Can you work these out from the model? Positions are in its coordinate system, mm. Face numbers are marked on the shaded views. A direction names the side the tool comes from. Round coordinates to 2 decimals unless told otherwise and drop trailing zeros. Write each loop counter-clockwise with the first axis right and the second up, starting at its lowest first coordinate (ties: lowest second). Pieces come first, ordered by that corner, then holes. Notation, with made-up numbers: (37.5, 54.5) - (51.5, 54.5) arc R24 ccw to (51.5, 69.5) - close; hole circle Ø7 at (43, -30). An arc over 180 degrees is marked (long way). One line per item, written item: value. Start each with the question number.
(1) Thinking about a two-plate mould opening in Z: for the marked faces 5, 6 and 7, which applies, +Z half, -Z half, draft (parallel to the pull), parting line (faces both ways), or undercut?
(2) I want a section at D-D on x = 3.75. List the corners of the cut face in (y, z) for me, plus the area to 3 significant figures.
(3) On a 3-axis mill with a long thin cutter (end or side, diameter ignored), from which of +Z, -Z, +X, -X, +Y, -Y can I reach the whole of each face in a straight line? I mean the marked faces 1, 2, 3 and 4. Say none if no direction works.
(4) I want a section at B-B on y = 7.5. List the corners of the cut face in (x, z) for me.
(5) I'm going to push flat-ended pins straight in: pin 1 Ø2 at (x, z) = (0.5, 3) entering from -Y; pin 2 Ø4.5 at (y, z) = (6, 6) entering from -X; pin 3 Ø3 at (x, z) = (10, 7) entering from +Y; pin 4 Ø1.5 at (x, y) = (-2.5, 1.5) entering from +Z. Where does each tip first touch, or does it pass through?
(6) I want a section at A-A on z = 5.75. List the corners of the cut face in (x, y) for me.
(7) If I drill on L1, parallel to X at y = 1.8, z = 5.75; L2, parallel to Z at x = 12, y = 1.8; L3, parallel to X at y = 4, z = 4.75, over which ranges is the centre line in solid material (lowest first)? Write a range as from..to.
(8) I want a section at C-C on z = 10.5. List the corners of the cut face in (x, y) for me.
from build123d import *

# Parameters (mm, degrees)
BOSS_EXTRUDE1_DEPTH = 13.5
SKETCH2_W           = 8
SKETCH2_H           = 8.5
BOSS_EXTRUDE2_DEPTH = 2
SKETCH3_R           = 1.65
BOSS_EXTRUDE3_DEPTH = 3


with BuildPart() as part:
    # Sketch1 → Boss-Extrude1 (new body)
    with BuildSketch(Plane.XY):
        Polygon((0, 0), (0, 8.5), (3, 8.5), (3, 3), (5, 3), (5, 8.5), (8, 8.5), (8, 0), align=None)
    extrude(amount=BOSS_EXTRUDE1_DEPTH)

    # Sketch2 → Boss-Extrude2 (add)
    with BuildSketch(Plane(origin=(0, 0, 0), x_dir=(-1, 0, 0), z_dir=(0, 0, -1))):
        with Locations((-4, 4.25)):
            Rectangle(SKETCH2_W, SKETCH2_H)
    extrude(amount=BOSS_EXTRUDE2_DEPTH)

    # Sketch3 → Boss-Extrude3 (add)
    with BuildSketch(Plane(origin=(0, 0, 0), x_dir=(1, 0, 0), z_dir=(0, 1, 0))):
        with BuildLine():
            Line((0, -2.75), (-4, -2.75))
            ThreePointArc((-4, -2.75), (-7, -5.75), (-4, -8.75))
            Line((-4, -8.75), (0, -8.75))
            Line((0, -8.75), (0, -2.75))
        make_face()
        with Locations((-4, -5.75)):
            Circle(SKETCH3_R, mode=Mode.SUBTRACT)
        with BuildLine():
            Line((8, -2.75), (12, -2.75))
            ThreePointArc((12, -2.75), (15, -5.75), (12, -8.75))
            Line((12, -8.75), (8, -8.75))
            Line((8, -8.75), (8, -2.75))
        make_face()
        with Locations((12, -5.75)):
            Circle(SKETCH3_R, mode=Mode.SUBTRACT)
    extrude(amount=BOSS_EXTRUDE3_DEPTH)


solid = part.part
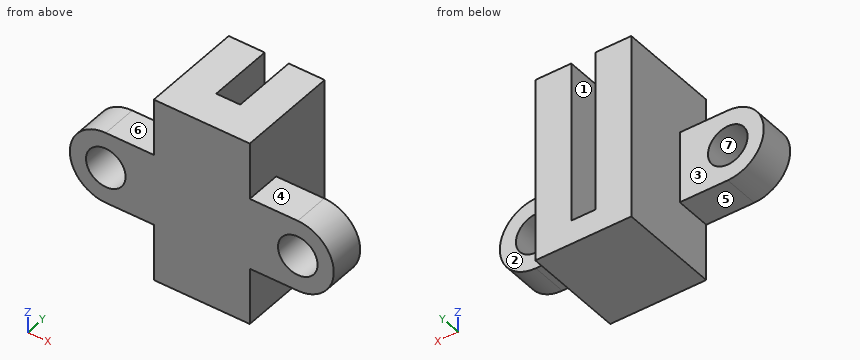
Established:
1. face 5: -Z half
1. face 6: +Z half
1. face 7: undercut
2. outline: (0, -2) - (8.5, -2) - (8.5, 0) - (3, 0) - (3, 13.5) - (0, 13.5) - close
2. area: 57.5 mm2
3. face 1: +Z, +Y
3. face 2: +Z, -Z, +X, +Y
3. face 3: +Z, -Z, -X, +Y
3. face 4: +Z, +X, +Y, -Y
4. outline: (0, -2) - (8, -2) - (8, 13.5) - (5, 13.5) - (5, 0) - (3, 0) - (3, 13.5) - (0, 13.5) - close
5. pin 1: y = 0
5. pin 2: x = 0
5. pin 3: y = 3
5. pin 4: z = 8.75
6. outline: (-7, 0) - (-5.65, 0) - (-5.65, 3) - (-7, 3) - close; (-2.35, 0) - (10.35, 0) - (10.35, 3) - (8, 3) - (8, 8.5) - (5, 8.5) - (5, 3) - (3, 3) - (3, 8.5) - (0, 8.5) - (0, 3) - (-2.35, 3) - close; (13.65, 0) - (15, 0) - (15, 3) - (13.65, 3) - close
7. L1: -7..-5.65, -2.35..10.35, 13.65..15
7. L2: 2.75..4.1, 7.4..8.75
7. L3: 0..3, 5..8
8. outline: (0, 0) - (8, 0) - (8, 8.5) - (5, 8.5) - (5, 3) - (3, 3) - (3, 8.5) - (0, 8.5) - close
